from build123d import *

# Parameters (mm, degrees)
F0_R      = 15.45
F0_R_2    = 12.25
F1_DEPTH  = 20
F2_W      = 70
F2_H      = 57
F3_DEPTH  = 2
F4_W      = 70
F4_H      = 25
F5_DEPTH  = 2
F6_W      = 70
F6_H      = 25
F7_DEPTH  = 2
F10_D     = 6
F11_W     = 61
F11_H     = 2
F12_DEPTH = 30
F14_DEPTH = 30


# Not quite as in the source:
# - a fillet or chamfer that OpenCascade refuses, or shapes differently, is made with other operations: its cross-section is extruded or revolved along the edge and cut away or added


with BuildPart() as f1:
    # F0 (on Top) → F1 (new body)
    with BuildSketch(Plane.XY):
        Circle(F0_R)
        Circle(F0_R_2, mode=Mode.SUBTRACT)
    extrude(amount=F1_DEPTH)

    # F2 (on face) → F3 (join)
    with BuildSketch(Plane.XY.offset(20)):
        Rectangle(F2_W, F2_H)
    extrude(amount=F3_DEPTH)

    # F4 (on face) → F5 (join)
    with BuildSketch(Plane.XZ.offset(28.5)):
        with Locations((0, 32.5)):
            Rectangle(F4_W, F4_H)
    extrude(amount=F5_DEPTH)

    # F6 (on face) → F7 (join)
    with BuildSketch(Plane(origin=(0, 28.5, 0), x_dir=(-1, 0, 0), z_dir=(0, 1, 0))):
        with Locations((0, 32.5)):
            Rectangle(F6_W, F6_H)
    extrude(amount=F7_DEPTH)

    # F8: chamfer of 7 on 3 edges, made by hand

    # F8_s1 → F8_t2 (revolve)
    with BuildSketch(Plane.XZ):
        Polygon((22.45, 20), (15.45, 13), (15.45, 20), align=None)
    revolve(axis=Axis((0, 0, 20), (0, 0, 1)))

    # F8_s3 → F8_t4 (revolve, cut)
    with BuildSketch(Plane.XZ):
        Polygon((15.45, 7), (8.45, 0), (15.45, 0), align=None)
    revolve(axis=Axis((0, 0, 0), (0, 0, 1)), mode=Mode.SUBTRACT)

    # F10 (through all)
    with Locations(Plane.XZ.offset(30.5)):
        with Locations((-23, 32.5), (23, 32.5)):
            Hole(F10_D / 2)

    # F11 (on face) → F12 (join)
    with BuildSketch(Plane(origin=(-35, 0, 0), x_dir=(0, -1, 0), z_dir=(-1, 0, 0))):
        with Locations((0, 21)):
            Rectangle(F11_W, F11_H)
    extrude(amount=F12_DEPTH)

    # F13 (on face) → F14 (join)
    with BuildSketch(Plane.YZ.offset(35)):
        Polygon((-30.5, 22), (-30.5, 20), (30.5, 20), (30.5, 22), (28.5, 22), (-28.5, 22), align=None)
    extrude(amount=F14_DEPTH)


solid = f1.part
Input: part model. Units: mm. Frame: model coordinates. A direction names the side the tool comes from. Round coordinates to 2 decimals unless told otherwise and drop trailing zeros. Write each loop counter-clockwise with the first axis right and the second up, starting at its lowest first coordinate (ties: lowest second). Pieces come first, ordered by that corner, then holes.
1) Cut plane A-A (z = 25.5). Return the cut outline in (x, y), then the cut area to 3 significant figures.
2) Cut plane C-C (x = 0). Return the cut outline in (y, z).
3) Draft query along Z for faces 4 (the cylindrical face through (-20.79, -29.49, 34.53)), 5 (the flat face through (-15, 20, 20)), 6 (the cylindrical face through (25.21, -29.49, 34.53)), 7 (the cylindrical face through (6.586, 10.329, 11.787)). Return one class per face: pulls with the +Z half, pulls with the -Z half, needs draft (parallel to the pull), parting line crosses it, or undercut.
4) Contact query for flat-ended pins moving along their axis: P1, Ø1.6, axis at y = 29.5, z = 28, coming from the +X side; P2, Ø1.6, axis at y = 29, z = 31.5, coming from the -X side; P3, Ø10, axis at y = 10, z = 12.5, coming from the +X side. Output: stop coordinate, or through.
5) Ray query, L1, parallel to X at y = 29, z = 32; L2, parallel to Y at x = -22, z = 27.5; L3, parallel to Y at x = 0, z = 13. Return the intervals inside material, ascending.
6) Cut plane D-D (z = 32.5). Return the cut outline in (x, y).
7) Cut plane B-B (y = 0). Return the cut outline in (x, z).
8) Reachability of faces 1 (the cylindrical face through (25.21, 29.51, 34.53)), 2 (the flat face through (0, -28.5, 34)), 3 (the cylindrical face through (-12.26, -9.4, 9.96)) from +Z, -Z, +X, -X, +Y, -Y: full face, straight path, thin tool, end or side. Return the list, or none.
Geometry says:
1. outline: (-35, -30.5) - (35, -30.5) - (35, -28.5) - (-35, -28.5) - close; (-35, 28.5) - (35, 28.5) - (35, 30.5) - (-35, 30.5) - close
1. area: 280 mm2
2. outline: (-30.5, 20) - (-22.45, 20) - (-15.45, 13) - (-15.45, 7) - (-12.25, 3.8) - (-12.25, 20) - (12.25, 20) - (12.25, 3.8) - (15.45, 7) - (15.45, 13) - (22.45, 20) - (30.5, 20) - (30.5, 45) - (28.5, 45) - (28.5, 22) - (-28.5, 22) - (-28.5, 45) - (-30.5, 45) - close
3. face 4: undercut
3. face 5: pulls with the -Z half
3. face 6: undercut
3. face 7: needs draft
4. P1: stops at x = 35
4. P2: stops at x = -35
4. P3: stops at x = 17.82
5. L1: x = -35 to -25.96, -20.04 to 20.04, 25.96 to 35
5. L2: y = -30.5 to -28.5, 28.5 to 30.5
5. L3: y = -15.45 to -12.25, 12.25 to 15.45
6. outline: (-35, -30.5) - (-26, -30.5) - (-26, -28.5) - (-35, -28.5) - close; (-35, 28.5) - (-26, 28.5) - (-26, 30.5) - (-35, 30.5) - close; (-20, -30.5) - (20, -30.5) - (20, -28.5) - (-20, -28.5) - close; (-20, 28.5) - (20, 28.5) - (20, 30.5) - (-20, 30.5) - close; (26, -30.5) - (35, -30.5) - (35, -28.5) - (26, -28.5) - close; (26, 28.5) - (35, 28.5) - (35, 30.5) - (26, 30.5) - close
7. outline: (-65, 20) - (-22.45, 20) - (-15.45, 13) - (-15.45, 7) - (-12.25, 3.8) - (-12.25, 20) - (12.25, 20) - (12.25, 3.8) - (15.45, 7) - (15.45, 13) - (22.45, 20) - (65, 20) - (65, 22) - (-65, 22) - close
8. face 1: +Y, -Y
8. face 2: +Z, +X, -X
8. face 3: -Z
